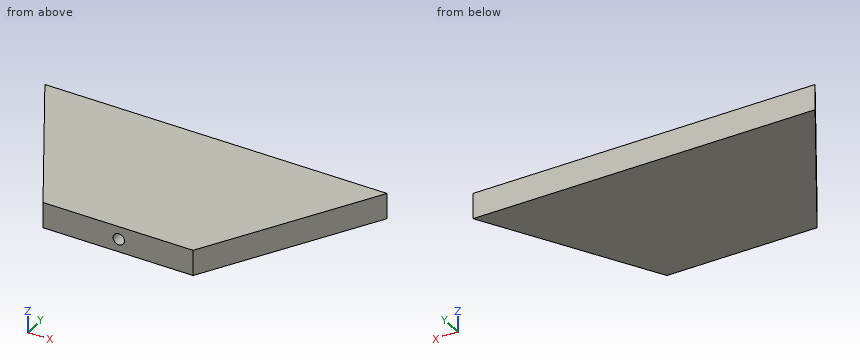
from build123d import *

# Parameters (mm, degrees)
BOSS_EXTRUDE1_DEPTH = 4
SKETCH6_R           = 1.75
CUT_EXTRUDE1_DEPTH  = 5


with BuildPart() as part:
    # Sketch5 → Boss-Extrude1 (new, symmetric)
    with BuildSketch(Plane.XY):
        Polygon((-52.571031757, -370.671309458), (53.31747051, -370.671309458), (22.981500363, -421.073600557), (-23.471255423, -421.073600557), align=None)
    extrude(amount=BOSS_EXTRUDE1_DEPTH, both=True)

    # Sketch6 → Cut-Extrude1 (cut)
    with BuildSketch(Plane.XZ.offset(421.073600557)):
        with Locations(Location((0, 0, 0), (0, 0, 270))):
            Circle(SKETCH6_R)
    extrude(amount=-CUT_EXTRUDE1_DEPTH, mode=Mode.SUBTRACT)


solid = part.part
CAD build for the part. Positions are in the model's coordinates, mm. Round coordinates to 2 decimals unless told otherwise and drop trailing zeros. Write each loop counter-clockwise with the first axis right and the second up, starting at its lowest first coordinate (ties: lowest second). Pieces come first, ordered by that corner, then holes.
(1) Drop flat-ended pins along their axis: P1, Ø12, axis at x = -41.5, y = -407, coming from the -Z side; P2, Ø1.8, axis at x = -0.5, z = 0, coming from the -Y side. Give the stop position or say it passes through.
(2) Slice it at B-B, the plane z = 0. Write the cut outline in (x, y).
(3) Probe line 1 along X through (y, z) = (-416.5, 1.25); line 2 along X through (y, z) = (-419.8, 0); line 3 along X through (y, z) = (-401.5, 3). List the from-to ranges inside material, lowest first.
(4) Slice it at D-D, the plane y = -397. Write the cut outline in (x, z).
(5) Slice it at A-A, the plane x = 0. Write the cut outline in (y, z), and give its area (3 significant figures).
(6) Slice it at C-C, the plane y = -409. Write the cut outline in (x, z).
From the geometry:
1. P1: passes through
1. P2: stops at y = -416.07
2. outline: (-52.57, -370.67) - (-23.47, -421.07) - (-1.75, -421.07) - (-1.75, -416.07) - (1.75, -416.07) - (1.75, -421.07) - (22.98, -421.07) - (53.32, -370.67) - close
3. line 1: x = -26.11 to -1.22, 1.22 to 25.73
3. line 2: x = -24.21 to -1.75, 1.75 to 23.75
3. line 3: x = -34.77 to 34.76
4. outline: (-37.37, -4) - (37.47, -4) - (37.47, 4) - (-37.37, 4) - close
5. outline: (-421.07, -4) - (-370.67, -4) - (-370.67, 4) - (-421.07, 4) - (-421.07, 1.75) - (-416.07, 1.75) - (-416.07, -1.75) - (-421.07, -1.75) - close
5. area: 386 mm2
6. outline: (-30.44, -4) - (30.25, -4) - (30.25, 4) - (-30.44, 4) - close
